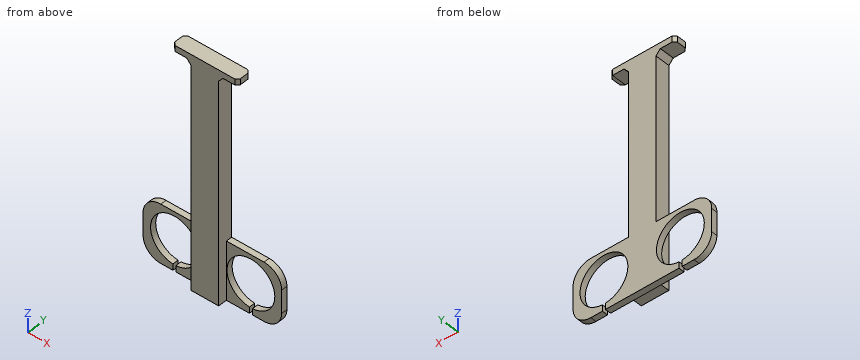
from build123d import *

# Parameters (mm, degrees)
F1_DEPTH = 2
F0_W     = 1.9
F0_H     = 55.0951848962
F0_W_2   = 3
F0_H_2   = 8.0191061349
F0_W_3   = 1.0669481622
F0_H_3   = 2
F0_H_4   = 17.6764619537
F0_H_5   = 2.0183531501
F2_DEPTH = 5
F3_SIZE  = 1


with BuildPart() as f1:
    # F0 (on Front) → F1 (new body)
    with BuildSketch(Plane.XZ):
        with BuildLine():
            Line((-5.2732866119, -11.4232450724), (-5.2732866119, 6.2532168813))
            Line((-5.2732866119, 6.2532168813), (-18.1692923009, 6.2532168813))
            ThreePointArc((-18.1692923009, 6.2532168813), (-22.4119329881, 4.4958575684), (-24.1692923009, 0.2532168813))
            Line((-24.1692923009, 0.2532168813), (-24.1692923009, -7.474217616))
            ThreePointArc((-24.1692923009, -7.474217616), (-22.4119329881, -11.7168583031), (-18.1692923009, -13.474217616))
            Line((-18.1692923009, -13.474217616), (-14.0744003764, -13.474217616))
            Line((-14.0744003764, -13.474217616), (-14.0744003764, -11.3696444416))
            ThreePointArc((-14.0744003764, -11.3696444416), (-13.5321325059, 4.8135476182), (-13.0744003764, -11.3722560686))
            Line((-13.0744003764, -11.3722560686), (-13.0744003764, -13.474217616))
            Line((-13.0744003764, -13.474217616), (11.8678271526, -13.474217616))
            Line((11.8678271526, -13.474217616), (11.8678271526, -11.3722560686))
            ThreePointArc((11.8678271526, -11.3722560686), (12.3255592821, 4.8135476182), (12.8678271526, -11.3696444416))
            Line((12.8678271526, -11.3696444416), (12.8678271526, -13.474217616))
            Line((12.8678271526, -13.474217616), (16.7931831032, -13.474217616))
            ThreePointArc((16.7931831032, -13.474217616), (21.0358237903, -11.7168583031), (22.7931831032, -7.474217616))
            Line((22.7931831032, -7.474217616), (22.7931831032, 0.2532168813))
            ThreePointArc((22.7931831032, 0.2532168813), (21.0358237903, 4.4958575684), (16.7931831032, 6.2532168813))
            Line((16.7931831032, 6.2532168813), (4.0667133881, 6.2532168813))
            Line((4.0667133881, 6.2532168813), (4.0667133881, -11.4232450724))
            Line((4.0667133881, -11.4232450724), (4.0667133881, -13.4415982225))
            Line((4.0667133881, -13.4415982225), (2.1667133881, -13.4415982225))
            Line((2.1667133881, -13.4415982225), (-3.3732866119, -13.4415982225))
            Line((-3.3732866119, -13.4415982225), (-5.2732866119, -13.4415982225))
            Line((-5.2732866119, -13.4415982225), (-5.2732866119, -11.4232450724))
        make_face()
    extrude(amount=F1_DEPTH)

    # F0 (on Front) → F2 (join)
    with BuildSketch(Plane.XZ):
        with Locations((-4.3232866119, 33.8008093294)):
            Rectangle(F0_W, F0_H)
        Polygon((-2.1032866119, 61.3484017775), (-3.3732866119, 61.3484017775), (-3.3732866119, 6.2532168813), (2.1667133881, 6.2532168813), (2.1667133881, 61.3484017775), (0.8967133881, 61.3484017775), (0.8967133881, 53.3292956426), (-2.1032866119, 53.3292956426), align=None)
        with Locations((3.1167133881, 33.8008093294)):
            Rectangle(F0_W, F0_H)
        with Locations((-0.6032866119, 57.3388487101)):
            Rectangle(F0_W_2, F0_H_2)
        Polygon((-6.7575482038, 62.9888176918), (-5.2732866119, 61.3484017775), (-3.3732866119, 61.3484017775), (-2.1032866119, 61.3484017775), (0.8967133881, 61.3484017775), (2.1667133881, 61.3484017775), (4.0667133881, 61.3484017775), (5.55097498, 62.9888176918), align=None)
        with Locations((-11.1823320082, 63.9888176918)):
            Rectangle(F0_W_3, F0_H_3)
        Polygon((9.4422847033, 64.9888176918), (9.4422847033, 62.9888176918), (10.5092328655, 62.9867687821), (10.5092328655, 64.9888176918), align=None)
        Polygon((-10.6488579271, 62.9888176918), (-6.7575482038, 62.9888176918), (5.55097498, 62.9888176918), (9.4422847033, 62.9888176918), (9.4422847033, 64.9888176918), (-10.6488579271, 64.9888176918), align=None)
        with Locations((-4.3232866119, -2.5850140955)):
            Rectangle(F0_W, F0_H_4)
        Polygon((2.1667133881, 6.2532168813), (-3.3732866119, 6.2532168813), (-3.3732866119, -11.4232450724), (-3.3732866119, -13.4415982225), (2.1667133881, -13.4415982225), (2.1667133881, -11.4232450724), align=None)
        with Locations((3.1167133881, -2.5850140955)):
            Rectangle(F0_W, F0_H_4)
        with Locations((-4.3232866119, -12.4324216474)):
            Rectangle(F0_W, F0_H_5)
        with Locations((3.1167133881, -12.4324216474)):
            Rectangle(F0_W, F0_H_5)
    extrude(amount=F2_DEPTH)

    # F3
    f3_edges = [f1.edges().sort_by_distance(p)[0] for p in [
        (10.509233, 0, 63.987793),
        (10.509233, -5, 63.987793),
        (-11.715806, -5, 63.988818),
        (-11.715806, 0, 63.988818),
    ]]
    chamfer(f3_edges, length=F3_SIZE)


solid = f1.part
Design review of the part built by this model. Coordinates are the model's own, in mm. Round coordinates to 2 decimals unless told otherwise and drop trailing zeros. Write each loop counter-clockwise with the first axis right and the second up, starting at its lowest first coordinate (ties: lowest second). Pieces come first, ordered by that corner, then holes. Notation, with made-up numbers: (-26.5, -12.5) - (-13.5, -12.5) arc R13 cw to (-13.5, 11.5) - close; hole circle Ø6 at (-26.5, 25.5). An arc over 180 degrees is marked (long way). Return JSON: item names as keys, results as strings. Group by question number.
Item 1: We need section C-C on y = -3.2. Write out the cut boundary in (x, z), and give its area (3 significant figures).
Item 2: For probe 1 along Z at (x, y) = (-10, -0.4); probe 2 along Z at (x, y) = (7.5, -1.8); probe 3 along X at (y, z) = (-0.55, -2), list the stretches that pass through material, from the lowest coordinate up. Write a range as [from, to].
Item 3: We need section A-A on x = 7.5. Write out the cut boundary in (y, z), and give its area (3 significant figures).
Item 4: We need section D-D on z = 51. Write out the cut boundary in (x, y).
Item 5: We need section B-B on z = -2.5. Write out the cut boundary in (x, y), and give its area (3 significant figures).
Item 6: Insertion check: P1, Ø1.6, axis at y = -0.5, z = -13, coming from the +X side; P2, Ø0.6, axis at y = -0.5, z = -12, coming from the -X side; P3, Ø0.6, axis at y = -3, z = 64, coming from the -X side. Each pin has a flat end and moves straight along its axis. Give the tip position at first contact, or say it passes through.
Model answer:
{
 "1": {"outline": "(-11.72, 62.99) - (-6.76, 62.99) - (-5.27, 61.35) - (-5.27, -13.44) - (4.07, -13.44) - (4.07, 61.35) - (5.55, 62.99) - (9.44, 62.99) - (10.51, 62.99) - (10.51, 64.99) - (-11.72, 64.99) - close", "area": "761 mm²"},
 "2": {"probe 1": "z = [-13.47, -10.57], [3.99, 6.25], [62.99, 64.99]", "probe 2": "z = [-13.47, -9.78], [3.2, 6.25], [62.99, 64.99]", "probe 3": "x = [-24.17, -21.55], [-5.56, 4.35], [20.34, 22.79]"},
 "3": {"outline": "(-5, 62.99) - (0, 62.99) - (0, 64.99) - (-5, 64.99) - close; (-2, -13.47) - (0, -13.47) - (0, -9.78) - (-2, -9.78) - close; (-2, 3.2) - (0, 3.2) - (0, 6.25) - (-2, 6.25) - close", "area": "23.5 mm²"},
 "4": {"outline": "(-5.27, -5) - (4.07, -5) - (4.07, 0) - (-5.27, 0) - close"},
 "5": {"outline": "(-24.17, -2) - (-21.62, -2) - (-21.62, 0) - (-24.17, 0) - close; (-5.49, -2) - (-5.27, -2) - (-5.27, -5) - (4.07, -5) - (4.07, -2) - (4.28, -2) - (4.28, 0) - (-5.49, 0) - close; (20.41, -2) - (22.79, -2) - (22.79, 0) - (20.41, 0) - close", "area": "57.5 mm²"},
 "6": {"P1": "stops at x = 20.49", "P2": "stops at x = -22.43", "P3": "stops at x = -11.72"}
}
